Input: part model. Units: mm. Frame: model coordinates. A direction names the side the tool comes from. Round coordinates to 2 decimals unless told otherwise and drop trailing zeros. Loops run counter-clockwise (first coordinate to the right, second up) from the corner with the lowest first, then second, coordinate; pieces in that order, holes last. Notation, with made-up numbers: (30, 33) - (88, 33) arc R11 ccw to (88, 48) - close; hole circle Ø7 at (68.25, -19.75). An arc over 180 degrees is marked (long way). One line per question, with ' | ' between items. Start each with the question number.
from build123d import *

# Parameters (mm, degrees)
SKETCH_1_R          = 2.75
EXTRUDE_1_DEPTH     = 9
SKETCH_6_R          = 4.25
CUT_EXTRUDE_3_DEPTH = 5
CHAMFER_2_SIZE      = 5
SKETCH_8_W          = 51
SKETCH_8_H          = 20
EXTRUDE_2_DEPTH     = 30
SKETCH_9_R          = 5.25
CUT_EXTRUDE_4_DEPTH = 60.245252974
CHAMFER_3_SIZE      = 10
CHAMFER_4_SIZE      = 5


with BuildPart() as part:
    # 草圖1 → 填料-伸長1 (new body)
    with BuildSketch(Plane.XY):
        Polygon((30, 23), (21, 23), (-21, 23), (-21, -23), (21, -23), (30, -23), align=None)
        with Locations((0, 17)):
            Circle(SKETCH_1_R, mode=Mode.SUBTRACT)
        with Locations((20, 17)):
            Circle(SKETCH_1_R, mode=Mode.SUBTRACT)
        with Locations((20, -17)):
            Circle(SKETCH_1_R, mode=Mode.SUBTRACT)
        with Locations((0, -17)):
            Circle(SKETCH_1_R, mode=Mode.SUBTRACT)
    extrude(amount=EXTRUDE_1_DEPTH)

    # 草圖6 → 除料-伸長3 (cut)
    with BuildSketch(Plane.XY.offset(9)):
        with Locations((0, 17)):
            Circle(SKETCH_6_R)
        with Locations((20, 17)):
            Circle(SKETCH_6_R)
        with Locations((20, -17)):
            Circle(SKETCH_6_R)
        with Locations((0, -17)):
            Circle(SKETCH_6_R)
    extrude(amount=-CUT_EXTRUDE_3_DEPTH, mode=Mode.SUBTRACT)

    # 導角2
    chamfer_2_edges = [part.edges().sort_by_distance(p)[0] for p in [
        (-21, 23, 4.5),
        (30, 23, 4.5),
        (30, -23, 4.5),
        (-21, -23, 4.5),
    ]]
    chamfer(chamfer_2_edges, length=CHAMFER_2_SIZE)

    # 草圖8 → 填料-伸長2 (add)
    with BuildSketch(Plane.XY.offset(9)):
        with Locations((4.5, 0)):
            Rectangle(SKETCH_8_W, SKETCH_8_H)
    extrude(amount=EXTRUDE_2_DEPTH)

    # 草圖9 → 除料-伸長4 (cut, through all)
    with BuildSketch(Plane(origin=(0, 10, 0), x_dir=(1, 0, 0), z_dir=(0, 1, 0))):
        with Locations(Location((0, -30, 0), (0, 0, 180))):
            Circle(SKETCH_9_R)
    extrude(amount=-CUT_EXTRUDE_4_DEPTH, mode=Mode.SUBTRACT)

    # 導角3
    chamfer_3_edges = [part.edges().sort_by_distance(p)[0] for p in [
        (-21, 0, 39),
        (30, 0, 39),
    ]]
    chamfer(chamfer_3_edges, length=CHAMFER_3_SIZE)

    # 導角4
    # the kernel refuses this chamfer: 5 mm, written as the material it adds along each edge
    with BuildSketch(Plane(origin=(-21, -10, 9), x_dir=(0, 0.027495876610586317, 0.9996219169112968), z_dir=(1, 0, 0))) as chamfer_4_piece_1_section:
        Polygon((CHAMFER_4_SIZE * 0.999621916911, CHAMFER_4_SIZE * 0.0274958766106), (-CHAMFER_4_SIZE * 0.0274958766106, CHAMFER_4_SIZE * 0.999621916911), (0, 0), align=None)
    chamfer_4_piece_1 = extrude(amount=51, mode=Mode.PRIVATE)
    chamfer_4_piece_1 = chamfer_4_piece_1 - Plane(origin=(0, -17, 10.693214972), x_dir=(1, 0, 0), z_dir=(0, 0, 1)) * Cylinder(4.25, 122, mode=Mode.PRIVATE)
    chamfer_4_piece_1 = chamfer_4_piece_1 - Plane(origin=(20, -17, 10.693214972), x_dir=(1, 0, 0), z_dir=(0, 0, 1)) * Cylinder(4.25, 122, mode=Mode.PRIVATE)
    add(chamfer_4_piece_1)
    with BuildSketch(Plane(origin=(30, 10, 9), x_dir=(0, -0.027495876610586317, 0.9996219169112968), z_dir=(-1, 0, 0))) as chamfer_4_piece_2_section:
        Polygon((CHAMFER_4_SIZE * 0.999621916911, CHAMFER_4_SIZE * 0.0274958766106), (-CHAMFER_4_SIZE * 0.0274958766106, CHAMFER_4_SIZE * 0.999621916911), (0, 0), align=None)
    chamfer_4_piece_2 = extrude(amount=51, mode=Mode.PRIVATE)
    chamfer_4_piece_2 = chamfer_4_piece_2 - Plane(origin=(0, 17, 10.693214972), x_dir=(1, 0, 0), z_dir=(0, 0, 1)) * Cylinder(4.25, 122, mode=Mode.PRIVATE)
    chamfer_4_piece_2 = chamfer_4_piece_2 - Plane(origin=(20, 17, 10.693214972), x_dir=(1, 0, 0), z_dir=(0, 0, 1)) * Cylinder(4.25, 122, mode=Mode.PRIVATE)
    add(chamfer_4_piece_2)


solid = part.part
(1) Pin query (flat end, axial travel): P1, Ø6.5, axis at x = 20, y = 17, coming from the +Z side; P2, Ø2.5, axis at x = -3.5, y = 18.5, coming from the +Z side; P3, Ø2, axis at x = 11.5, z = 17, coming from the +Y side. Return the tip coordinate at first contact, or that it passes through.
(2) Section B-B, the plane z = 30. Output: boundary loops of the cut face in (x, y).
(3) Section A-A, the plane y = 17. Output: boundary loops of the cut face in (x, z), plus the area to 3 significant figures.
(4) Section D-D, the plane z = 8. Output: boundary loops of the cut face in (x, y), plus the area to 3 significant figures.
(5) Pull-direction query (Y, two-part tool) for faces 4 (the face through (4, -12, 12)), 5 (the face through (-0.92, 12.85, 7.02)), 6 (the face through (4, 19, 9)), 7 (the face through (0, 14, 4)); classes: released by +Y, released by -Y, zero draft, split by the parting line, or undercut.
(6) Line query: line 1 along X through (y, z) = (-17, 8); line 2 along Y through (x, z) = (0, 2); line 3 along Y through (x, z) = (20, 6). Output: solid intervals per line, ascending. Write a range as from..to.
(7) Section C-C, the plane x = 0. Output: boundary loops of the cut face in (y, z), plus the area to 3 significant figures.
(8) Reachability of faces 1 (the face through (20, 14, 4)), 2 (the face through (28, 20, 4)), 3 (the face through (4, -10, 26)) from +Z, -Z, +X, -X, +Y, -Y: full face, straight path, thin tool, end or side. Return the list, or none.
Derived:
1) P1: stops at z = 4 | P2: stops at z = 9 | P3: stops at y = 10
2) outline: (-20, -10) - (-5.25, -10) - (-5.25, 10) - (-20, 10) - close; (5.25, -10) - (29, -10) - (29, 10) - (5.25, 10) - close
3) outline: (-21, 0) - (-2.75, 0) - (-2.75, 4) - (-4.25, 4) - (-4.25, 9) - (-21, 9) - close; (2.75, 0) - (17.25, 0) - (17.25, 4) - (15.75, 4) - (15.75, 9) - (4.25, 9) - (4.25, 4) - (2.75, 4) - close; (22.75, 0) - (30, 0) - (30, 9) - (24.25, 9) - (24.25, 4) - (22.75, 4) - close | area: 330 mm²
4) outline: (-21, -18) - (-16, -23) - (25, -23) - (30, -18) - (30, 18) - (25, 23) - (-16, 23) - (-21, 18) - close; hole circle Ø8.5 at (0, -17); hole circle Ø8.5 at (0, 17); hole circle Ø8.5 at (20, -17); hole circle Ø8.5 at (20, 17) | area: 2,070 mm²
5) face 4: released by -Y | face 5: undercut | face 6: zero draft | face 7: undercut
6) line 1: x = -21..-4.25, 4.25..15.75, 24.25..30 | line 2: y = -23..-19.75, -14.25..14.25, 19.75..23 | line 3: y = -23..-21.25, -12.75..12.75, 21.25..23
7) outline: (-23, 0) - (-19.75, 0) - (-19.75, 4) - (-21.25, 4) - (-21.25, 9) - (-23, 9) - close; (-14.25, 0) - (14.25, 0) - (14.25, 4) - (12.75, 4) - (12.75, 11.25) - (10, 14) - (10, 24.75) - (-10, 24.75) - (-10, 14) - (-12.75, 11.25) - (-12.75, 4) - (-14.25, 4) - close; (-10, 35.25) - (10, 35.25) - (10, 39) - (-10, 39) - close; (19.75, 0) - (23, 0) - (23, 9) - (21.25, 9) - (21.25, 4) - (19.75, 4) - close | area: 695 mm²
8) face 1: +Z | face 2: +Z, -Z, +X, +Y | face 3: +Z, +X, -X, -Y
